```python
from build123d import *

# Parameters (mm, degrees)
CUT_EXTRUDE_1_DEPTH = 1.5
FILLET_1_R          = 0.2
CHAMFER_1_SIZE      = 0.2


with BuildPart() as part:
    # 草图1 → 旋转1 (revolve)
    with BuildSketch(Plane.XY):
        Polygon((-5, 0), (-5, 1.8), (-3, 1.8), (-3, 1), (5, 1), (5, 0), align=None)
    revolve(axis=Axis((5, 0, 0), (-1, 0, 0)))

    # 草图2 → 切除-拉伸1 (cut)
    with BuildSketch(Plane.ZY.offset(5)):
        Polygon((0.866025404, 0), (0.433012702, 0.75), (-0.433012702, 0.75), (-0.866025404, 0), (-0.433012702, -0.75), (0.433012702, -0.75), align=None)
    extrude(amount=-CUT_EXTRUDE_1_DEPTH, mode=Mode.SUBTRACT)

    # 圆角1
    fillet_1_edges = [part.edges().sort_by_distance(p)[0] for p in [
        (-3, -1.8, 0),
        (-5, -1.8, 0),
    ]]
    fillet(fillet_1_edges, radius=FILLET_1_R)

    # 倒角1
    chamfer_1_edges = [part.edges().sort_by_distance(p)[0] for p in [
        (5, -1, 0),
    ]]
    chamfer(chamfer_1_edges, length=CHAMFER_1_SIZE)


solid = part.part
```
Part model, mm, in its own coordinate system. A direction names the side the tool comes from. Give positions to 0.01 mm unless a question says otherwise; leave off trailing zeros. Order: outer loops, then holes, each group sorted by start corner. A loop starts at its lowest first (then second) coordinate and runs counter-clockwise, first axis right, second up. Notation, with made-up numbers: M 20,-22 L 65,-22 A22 cw 65,11 Z; hole C -36.5,17.5 d1. An arc over 180 degrees is marked long. Use a Markdown table: item, result. Add a question column.
(1) Saw through at B-B, the plane z = 0. Give the cut face in (x, y), and give its area (3 significant figures).
(2) Mould opens along Z. For faces 1 (the face through (-3.5, 0, 0)), 2 (the face through (-3.989, 1.717, -0.541)), 3 (the face through (5, 0, 0)) say: +Z half, -Z half, draft (parallel to the pull), parting line (faces both ways), or undercut.
(3) 3-axis set-ups, long thin cutter, end or side, ignore diameter. For faces 4 (the face through (-5, -1, 1)), 5 (the face through (-4, -0.75, 0)), 6 (the face through (-3, -1, 1)): which of +Z, -Z, +X, -X, +Y, -Y reach the whole face in a straight line?
(4) Drop a flat-ended pin along its axis: P1, Ø2, axis at x = 1.5, y = 1, coming from the -Z side. Give the stop position or say it passes through.
(5) Saw through at A-A, the plane x = -3.75. Give the cut face in (y, z), and give its area (3 significant figures).
(6) Probe line 1 along X through (y, z) = (0.1, -0.7); line 2 along X through (y, z) = (1.35, -0.7); line 3 along Y through (x, z) = (-0.5, 0.9). List the from-to ranges inside material, lowest first. Write a range as [from, to].
(7) Saw through at C-C, the plane x = -1.75. Give the cut face in (y, z).
Answer key:
| question | item | result |
|---|---|---|
| 1 | outline | M -5,-1.6 A0.2 ccw -4.8,-1.8 L -3.2,-1.8 A0.2 ccw -3,-1.6 L -3,-1 L 4.8,-1 L 5,-0.8 L 5,0.8 L 4.8,1 L -3,1 L -3,1.6 A0.2 ccw -3.2,1.8 L -4.8,1.8 A0.2 ccw -5,1.6 L -5,0.75 L -3.5,0.75 L -3.5,-0.75 L -5,-0.75 Z |
| 1 | area | 20.9 mm^2 |
| 2 | face 1 | undercut |
| 2 | face 2 | parting line |
| 2 | face 3 | draft |
| 3 | face 4 | +Z, -Z, -X, +Y, -Y |
| 3 | face 5 | -X |
| 3 | face 6 | +X |
| 4 | P1 | z = -1 |
| 5 | outline | C 0,0 d3.6; hole M -0.75,-0.43 L 0,-0.87 L 0.75,-0.43 L 0.75,0.43 L 0,0.87 L -0.75,0.43 Z |
| 5 | area | 8.23 mm^2 |
| 6 | line 1 | [-3.5, 5] |
| 6 | line 2 | [-5, -3] |
| 6 | line 3 | [-0.44, 0.44] |
| 7 | outline | C 0,0 d2 |
